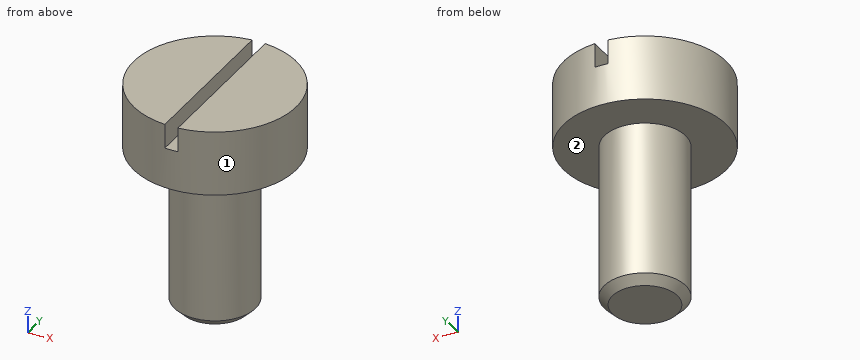
from build123d import *

# Parameters (mm, degrees)
SKETCH_1_R          = 2.5
EXTRUDE_1_DEPTH     = 10
SKETCH_2_R          = 5
EXTRUDE_2_DEPTH     = 4
SKETCH_3_W          = 0.8
SKETCH_3_H          = 11.405632212
CUT_EXTRUDE_1_DEPTH = 1.5
CHAMFER_1_SIZE      = 0.5


with BuildPart() as part:
    # Эскиз1 → Вытянуть1 (new body)
    with BuildSketch(Plane.XY):
        Circle(SKETCH_1_R)
    extrude(amount=EXTRUDE_1_DEPTH)

    # Эскиз2 → Вытянуть2 (add)
    with BuildSketch(Plane.XY.offset(10)):
        with Locations(Location((0, 0, 0), (0, 0, 94.588565736))):
            Circle(SKETCH_2_R)
    extrude(amount=EXTRUDE_2_DEPTH)

    # Эскиз3 → Вырез-Вытянуть1 (cut)
    with BuildSketch(Plane.XY.offset(14)):
        with Locations((0, 0.088759784)):
            Rectangle(SKETCH_3_W, SKETCH_3_H)
    extrude(amount=-CUT_EXTRUDE_1_DEPTH, mode=Mode.SUBTRACT)

    # Фаска1
    chamfer_1_edges = [part.edges().sort_by_distance(p)[0] for p in [
        (-2.5, 0, 0),
    ]]
    chamfer(chamfer_1_edges, length=CHAMFER_1_SIZE)


solid = part.part
Read the model definition and answer for the solid it produces. Units are mm, in the model's axes. Face numbers are marked on the shaded views. A direction names the side the tool comes from. Coordinates: 2 decimals unless noted, no trailing zeros. Order: outer loops, then holes, each group sorted by start corner. A loop starts at its lowest first (then second) coordinate and runs counter-clockwise, first axis right, second up. Notation, with made-up numbers: (-22, -25.5) -> (28, -25.5) arc R17 cw to (28, -7.5) -> close; hole circle Ø4 at (32, -16.75). An arc over 180 degrees is marked (long way). Answer as a JSON object with one key per item and string values.
1) A cutting plane is placed at C-C, the plane x = 0. Determine the outline of the cut face in (y, z).
Model answer:
{"outline": "(-5, 10) -> (-2.5, 10) -> (-2.5, 0.5) -> (-2, 0) -> (2, 0) -> (2.5, 0.5) -> (2.5, 10) -> (5, 10) -> (5, 12.5) -> (-5, 12.5) -> close"}
2) A cutting plane is placed at D-D, the plane z = 6.25. Determine the outline of the cut face in (x, y), plus the area to 3 significant figures.
Model answer:
{"outline": "circle Ø5 at (0, 0)", "area": "19.6 mm²"}
3) A cutting plane is placed at A-A, the plane y = 0. Determine the outline of the cut face in (x, z), plus the area to 4 significant figures.
Model answer:
{"outline": "(-5, 10) -> (-2.5, 10) -> (-2.5, 0.5) -> (-2, 0) -> (2, 0) -> (2.5, 0.5) -> (2.5, 10) -> (5, 10) -> (5, 14) -> (0.4, 14) -> (0.4, 12.5) -> (-0.4, 12.5) -> (-0.4, 14) -> (-5, 14) -> close", "area": "88.55 mm²"}
4) A tool of negligible diameter and unlimited length cuts with its end or side. For the marked faces 1 and 2, from which of +Z, -Z, +X, -X, +Y, -Y can it reach the whole face along a straight path? Write none if from no direction.
Model answer:
{"face 1": "+Z, -Z", "face 2": "-Z"}
5) Consider line 1 along Z through (x, y) = (2, 4.25); line 2 along Y through (x, z) = (0.75, 4.75); line 3 along Y through (x, z) = (0.5, 13). Determine where each line is inside the solid, lowest interval first. Write a range as from..to.
Model answer:
{"line 1": "z = 10..14", "line 2": "y = -2.38..2.38", "line 3": "y = -4.97..4.97"}
6) Each of these flat-tipped pins is pushed along its axis until it touches: pin 1 (1 mm diameter, centred on y = 2, z = 6.5, fed in from -X); pin 2 (1.2 mm diameter, centred on y = -2, z = 13.5, fed in from +X); pin 3 (6 mm diameter, centred on x = -2.5, z = 5.5, fed in from +Y). Where does it stop, or does it pass through?
Model answer:
{"pin 1": "stops at x = -2", "pin 2": "stops at x = 4.8", "pin 3": "stops at y = 2.5"}
